```python
from build123d import *

# Parameters (mm, degrees)
SKETCH2_R           = 1.75
SKETCH2_R_2         = 4
BOSS_EXTRUDE1_DEPTH = 5
SKETCH3_R           = 7.5
SKETCH3_R_2         = 4
BOSS_EXTRUDE2_DEPTH = 19
SKETCH4_R           = 2.8
CUT_EXTRUDE1_DEPTH  = 3


with BuildPart() as part:
    # Sketch2 → Boss-Extrude1 (new body)
    with BuildSketch(Plane.XY):
        Polygon((-8.964466094, 12.5), (8.964466094, 12.5), (12.5, 8.964466094), (12.5, -8.964466094), (8.964466094, -12.5), (-8.964466094, -12.5), (-12.5, -8.964466094), (-12.5, 8.964466094), align=None)
        with Locations((-8.485281374, 8.485281374)):
            Circle(SKETCH2_R, mode=Mode.SUBTRACT)
        with Locations((8.485281374, -8.485281374)):
            Circle(SKETCH2_R, mode=Mode.SUBTRACT)
        with Locations((8.485281374, 8.485281374)):
            Circle(SKETCH2_R, mode=Mode.SUBTRACT)
        with Locations((-8.485281374, -8.485281374)):
            Circle(SKETCH2_R, mode=Mode.SUBTRACT)
        Circle(SKETCH2_R_2, mode=Mode.SUBTRACT)
    extrude(amount=BOSS_EXTRUDE1_DEPTH)

    # Sketch3 → Boss-Extrude2 (add)
    with BuildSketch(Plane.XY.offset(5)):
        with Locations(Location((0, 0, 0), (0, 0, 180))):
            Circle(SKETCH3_R)
        Circle(SKETCH3_R_2, mode=Mode.SUBTRACT)
    extrude(amount=BOSS_EXTRUDE2_DEPTH)

    # Sketch4 → Cut-Extrude1 (cut)
    with BuildSketch(Plane(origin=(0, 0, 0), x_dir=(-1, 0, 0), z_dir=(0, 0, -1))):
        with Locations((-8.485281374, 8.485281374)):
            Circle(SKETCH4_R)
        with Locations((8.485281374, 8.485281374)):
            Circle(SKETCH4_R)
        with Locations((8.485281374, -8.485281374)):
            Circle(SKETCH4_R)
        with Locations((-8.485281374, -8.485281374)):
            Circle(SKETCH4_R)
    extrude(amount=-CUT_EXTRUDE1_DEPTH, mode=Mode.SUBTRACT)


solid = part.part
```
Can you work these out from the model? Positions are in its coordinate system, mm. A direction names the side the tool comes from. Coordinates: 2 decimals unless noted, no trailing zeros. Loops run counter-clockwise (first coordinate to the right, second up) from the corner with the lowest first, then second, coordinate; pieces in that order, holes last.
1) Which directions (+Z, -Z, +X, -X, +Y, -Y) give clear straight access to the entire face, cutting with the end or side of a thin tool? Please do faces 4 (the flat face through (7, 10, 3)), 5 (the flat face through (10.757, -10.707, 2.465)).
2) For pin 1 (4 mm diameter, centred on x = -7, z = 14, fed in from +Y); pin 2 (10 mm diameter, centred on x = 8.5, z = 12, fed in from +Y); pin 3 (5.5 mm diameter, centred on x = 8.49, y = 8.49, fed in from -Z), each with a flat end and sliding along its axis, tell me the tip position at first contact or that it passes through.
3) Imagine slicing it at A-A on x = 0. List the corners of the cut face in (y, z) for me.
4) I need wall thicknesses on probe 1 along Y at (x, z) = (6.75, 1.75); probe 2 along Y at (x, z) = (0, 10.75); probe 3 along Y at (x, z) = (9.75, 1.75). Which ranges of each line are inside material? Lowest first, please.
5) Imagine slicing it at D-D on z = 15.5. List the corners of the cut face in (x, y) for me, plus the area to 3 significant figures.
6) Imagine slicing it at C-C on y = 9.5. List the corners of the cut face in (x, z) for me, plus the area to 3 significant figures.
7) Thinking about a two-plate mould opening in Y: for faces 1 (the flat face through (0, -12.5, 2)), 2 (the flat face through (10, -10, 3)), 3 (the cylindrical face through (-4.032, -6.324, 14.367)), which applies, pulls with the +Y half, pulls with the -Y half, needs draft (parallel to the pull), parting line crosses it, or undercut?
Completed:
1. face 4: -Z
1. face 5: +Z, -Z, +X, -Y
2. pin 1: stops at y = 5.59
2. pin 2: stops at y = 6.63
2. pin 3: stops at z = 3
3. outline: (-12.5, 0) - (-4, 0) - (-4, 24) - (-7.5, 24) - (-7.5, 5) - (-12.5, 5) - close; (4, 0) - (12.5, 0) - (12.5, 5) - (7.5, 5) - (7.5, 24) - (4, 24) - close
4. probe 1: y = -12.5 to -10.68, -6.29 to 6.29, 10.68 to 12.5
4. probe 2: y = -7.5 to -4, 4 to 7.5
4. probe 3: y = -11.71 to -10.98, -5.99 to 5.99, 10.98 to 11.71
5. outline: circle Ø15 at (0, 0); hole circle Ø8 at (0, 0)
5. area: 126 mm2
6. outline: (-11.96, 0) - (-11.09, 0) - (-11.09, 3) - (-9.91, 3) - (-9.91, 5) - (-11.96, 5) - close; (-7.06, 3) - (-5.88, 3) - (-5.88, 0) - (5.88, 0) - (5.88, 3) - (7.06, 3) - (7.06, 5) - (-7.06, 5) - close; (9.91, 3) - (11.09, 3) - (11.09, 0) - (11.96, 0) - (11.96, 5) - (9.91, 5) - close
6. area: 76.9 mm2
7. face 1: pulls with the -Y half
7. face 2: undercut
7. face 3: parting line crosses it
